from build123d import *

# Parameters (mm, degrees)
F0_R     = 9.525
F1_DEPTH = 60.325
F2_R     = 4.167188
F3_DEPTH = 38.1
F4_R     = 4.960938
F5_DEPTH = 31.75


with BuildPart() as f1:
    # F0 (on Front) → F1 (new body, symmetric)
    with BuildSketch(Plane.XZ):
        Circle(F0_R)
    extrude(amount=F1_DEPTH, both=True)

    # F2 (on face) → F3 (cut)
    with BuildSketch(Plane.XZ.offset(60.325)):
        Circle(F2_R)
    extrude(amount=-F3_DEPTH, mode=Mode.SUBTRACT)

    # F4 (on face) → F5 (cut)
    with BuildSketch(Plane(origin=(0, 60.325, 0), x_dir=(-1, 0, 0), z_dir=(0, 1, 0))):
        Circle(F4_R)
    extrude(amount=-F5_DEPTH, mode=Mode.SUBTRACT)


solid = f1.part
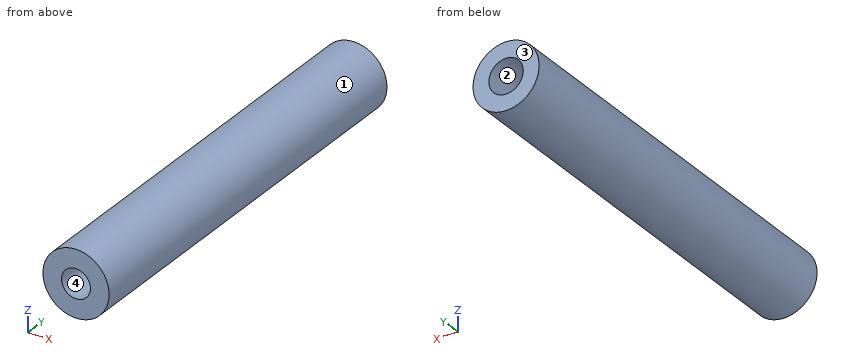
Input: part model. Units: mm. Frame: model coordinates. Face numbers are marked on the shaded views. Give positions to 0.01 mm unless a question says otherwise; leave off trailing zeros. Order: outer loops, then holes, each group sorted by start corner. A loop starts at its lowest first (then second) coordinate and runs counter-clockwise, first axis right, second up. Notation, with made-up numbers: M 10,10.5 L 16,10.5 A13 ccw 16,23.5 Z; hole C 74.25,59.25 d2. An arc over 180 degrees is marked long. Answer as a JSON object with one key per item and string values.
1. Ray query, line 1 (Z direction, x = 0.25, y = -23); line 2 (Z direction, x = 0, y = 39) (3 decimals); line 3 (X direction, y = 44.5, z = -2.5). Return the intervals inside material, ascending. Write a range as [from, to].
Result sheet:
{"line 1": "[-9.52, -4.16], [4.16, 9.52]", "line 2": "[-9.525, -4.961], [4.961, 9.525]", "line 3": "[-9.19, -4.28], [4.28, 9.19]"}
2. First-contact query: P1, Ø6, axis at y = 10, z = 4.5, coming from the -X side; P2, Ø8, axis at y = 7.5, z = -7.5, coming from the +X side; P3, Ø3, axis at x = -4, y = -35.5, coming from the -Z side. Flat tips, straight axial feed; report the tip coordinate or a pass-through.
Result sheet:
{"P1": "x = -9.41", "P2": "x = 8.86", "P3": "z = -9.19"}
3. Pull-direction query (Z, two-part tool) for the marked faces 1, 2, 3 and 4; classes: +Z half, -Z half, draft (parallel to the pull), parting line (faces both ways), or undercut.
Result sheet:
{"face 1": "parting line", "face 2": "undercut", "face 3": "draft", "face 4": "undercut"}
4. Cut plane B-B, the plane x = 0. Output: boundary loops of the cut face in (y, z) (3 decimals).
Result sheet:
{"outline": "M -60.325,-9.525 L 60.325,-9.525 L 60.325,-4.961 L 28.575,-4.961 L 28.575,4.961 L 60.325,4.961 L 60.325,9.525 L -60.325,9.525 L -60.325,4.167 L -22.225,4.167 L -22.225,-4.167 L -60.325,-4.167 Z"}
5. Cut plane A-A, the plane z = 0. Output: boundary loops of the cut face in (x, y) (3 decimals).
Result sheet:
{"outline": "M -9.525,-60.325 L -4.167,-60.325 L -4.167,-22.225 L 4.167,-22.225 L 4.167,-60.325 L 9.525,-60.325 L 9.525,60.325 L 4.961,60.325 L 4.961,28.575 L -4.961,28.575 L -4.961,60.325 L -9.525,60.325 Z"}
6. Cut plane D-D, the plane y = 17. Output: boundary loops of the cut face in (x, z) (3 decimals).
Result sheet:
{"outline": "C 0,0 d19.05"}
7. Cut plane C-C, the plane y = -36.5. Output: boundary loops of the cut face in (x, z) (3 decimals), and give its area (3 significant figures).
Result sheet:
{"outline": "C 0,0 d19.05; hole C 0,0 d8.334", "area": "230 mm²"}
